Verification items for this drawing (mm, ordinates from the low corner). Coordinates: 2 decimals unless noted, no trailing zeros. Loops run counter-clockwise (first coordinate to the right, second up) from the corner with the lowest first, then second, coordinate; pieces in that order, holes last. Notation, with made-up numbers: (-3, -37) - (27, -37) arc R30 ccw to (27, -12) - close; hole circle Ø10 at (35.25, 40.5). An arc over 180 degrees is marked (long way). One line per item, written item: value. Start each with the question number.
(1) Section check B-B (x = 1). Record the boundary of the cut face in (y, z) (1 decimal).
(2) Section check A-A (z = 1.75). Record the boundary of the cut face in (x, y).
(3) Draft check along X on the marked faces 1, 2, 3 and 4. Enter one of: +X half, -X half, draft (parallel to the pull), parting line (faces both ways), or undercut.
(4) Gauge pin test, flat end, axial feed: P1, Ø3.5, axis at x = 4, y = 4.62, coming from the -Z side. Record the tip position at first contact, or that the pin passes through.
(5) Thickness scan on probe 1 along Y at (x, z) = (3, 1.55) (1 decimal); probe 2 along Y at (x, z) = (7.25, 0.4) (1 decimal); probe 3 along Y at (x, z) = (1.25, 0.7). Record the ranges inside material, lowest first. Write a range as [from, to].
(6) Section check C-C (y = 1.5). Record the boundary of the cut face in (x, z), plus the area to 3 significant figures.
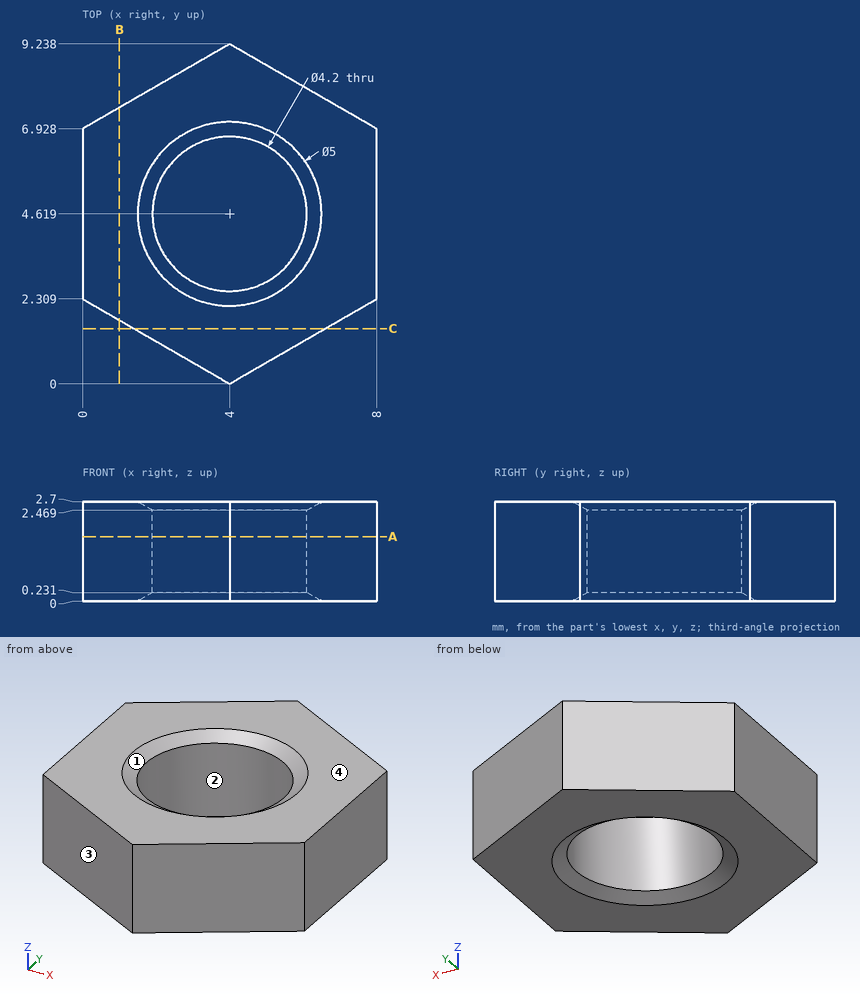
Responses:
1. outline: (1.7, 0) - (7.5, 0) - (7.5, 2.7) - (1.7, 2.7) - close
2. outline: (0, 2.31) - (4, 0) - (8, 2.31) - (8, 6.93) - (4, 9.24) - (0, 6.93) - close; hole circle Ø4.2 at (4, 4.62)
3. face 1: undercut
3. face 2: undercut
3. face 3: -X half
3. face 4: draft
4. P1: passes through
5. probe 1: y = [0.6, 2.8], [6.5, 8.7]
5. probe 2: y = [1.9, 7.4]
5. probe 3: y = [1.59, 7.65]
6. outline: (1.4, 0) - (6.6, 0) - (6.6, 2.7) - (1.4, 2.7) - close
6. area: 14.0 mm²
